from build123d import *

# Parameters (mm, degrees)
SKETCH1_W                      = 120
SKETCH1_H                      = 120
BOSS_EXTRUDE1_DEPTH            = 3
CUT_EXTRUDE1_REACH             = 5
CUT_EXTRUDE1_DIRECTION_2_DEPTH = 1
CUT_EXTRUDE2_REACH             = 5
SKETCH3_R                      = 2.75
SKETCH5_W                      = 124.8
SKETCH5_H                      = 124.8
SKETCH5_W_2                    = 120
SKETCH5_H_2                    = 120
BOSS_EXTRUDE2_DEPTH            = 28
SKETCH6_R                      = 1.65
CUT_EXTRUDE3_DEPTH             = 125.8
SKETCH7_W                      = 4
SKETCH7_H                      = 2
CUT_EXTRUDE4_DEPTH             = 125.8


with BuildPart() as part:
    # Sketch1 → Boss-Extrude1 (new body)
    with BuildSketch(Plane(origin=(0, 0, 0), x_dir=(1, 0, 0), z_dir=(0, 1, 0))):
        with Locations((60, 60)):
            Rectangle(SKETCH1_W, SKETCH1_H)
    extrude(amount=BOSS_EXTRUDE1_DEPTH)

    # Sketch2 → Cut-Extrude1 (cut, up to next)
    with BuildSketch(Plane(origin=(0, 3, 0), x_dir=(1, 0, 0), z_dir=(0, 1, 0)), mode=Mode.PRIVATE) as cut_extrude1_sk1:
        Polygon((15, 115), (57.5, 115), (57.5, 62.5), (5, 62.5), (5, 105), (15, 105), align=None)
    cut_extrude1_tool1 = extrude(cut_extrude1_sk1.sketch, amount=-CUT_EXTRUDE1_REACH, mode=Mode.PRIVATE) & part.part
    add(cut_extrude1_tool1.solids().sort_by_distance((32.05, 3, -87.95))[0], mode=Mode.SUBTRACT)
    # Sketch2 → Cut-Extrude1 (cut, up to next)
    with BuildSketch(Plane(origin=(0, 3, 0), x_dir=(1, 0, 0), z_dir=(0, 1, 0)), mode=Mode.PRIVATE) as cut_extrude1_sk2:
        Polygon((62.5, 5), (62.5, 57.5), (115, 57.5), (115, 15), (105, 15), (105, 5), align=None)
    cut_extrude1_tool2 = extrude(cut_extrude1_sk2.sketch, amount=-CUT_EXTRUDE1_REACH, mode=Mode.PRIVATE) & part.part
    add(cut_extrude1_tool2.solids().sort_by_distance((87.95, 3, -32.05))[0], mode=Mode.SUBTRACT)
    # Sketch2 → Cut-Extrude1 (cut, up to next)
    with BuildSketch(Plane(origin=(0, 3, 0), x_dir=(1, 0, 0), z_dir=(0, 1, 0)), mode=Mode.PRIVATE) as cut_extrude1_sk3:
        Polygon((15, 5), (57.5, 5), (57.5, 57.5), (5, 57.5), (5, 15), (15, 15), align=None)
    cut_extrude1_tool3 = extrude(cut_extrude1_sk3.sketch, amount=-CUT_EXTRUDE1_REACH, mode=Mode.PRIVATE) & part.part
    add(cut_extrude1_tool3.solids().sort_by_distance((32.05, 3, -32.05))[0], mode=Mode.SUBTRACT)
    # Sketch2 → Cut-Extrude1 (cut, up to next)
    with BuildSketch(Plane(origin=(0, 3, 0), x_dir=(1, 0, 0), z_dir=(0, 1, 0)), mode=Mode.PRIVATE) as cut_extrude1_sk4:
        Polygon((115, 62.5), (62.5, 62.5), (62.5, 115), (105, 115), (105, 105), (115, 105), align=None)
    cut_extrude1_tool4 = extrude(cut_extrude1_sk4.sketch, amount=-CUT_EXTRUDE1_REACH, mode=Mode.PRIVATE) & part.part
    add(cut_extrude1_tool4.solids().sort_by_distance((87.95, 3, -87.95))[0], mode=Mode.SUBTRACT)

    # Sketch2 → Cut-Extrude1 direction 2 (cut)
    with BuildSketch(Plane(origin=(0, 3, 0), x_dir=(1, 0, 0), z_dir=(0, 1, 0))):
        Polygon((15, 115), (57.5, 115), (57.5, 62.5), (5, 62.5), (5, 105), (15, 105), align=None)
        Polygon((62.5, 5), (62.5, 57.5), (115, 57.5), (115, 15), (105, 15), (105, 5), align=None)
        Polygon((15, 5), (57.5, 5), (57.5, 57.5), (5, 57.5), (5, 15), (15, 15), align=None)
        Polygon((115, 62.5), (62.5, 62.5), (62.5, 115), (105, 115), (105, 105), (115, 105), align=None)
    extrude(amount=CUT_EXTRUDE1_DIRECTION_2_DEPTH, mode=Mode.SUBTRACT)

    # Sketch3 → Cut-Extrude2 (cut, up to next)
    with BuildSketch(Plane(origin=(0, 3, 0), x_dir=(1, 0, 0), z_dir=(0, 1, 0)), mode=Mode.PRIVATE) as cut_extrude2_sk1:
        with Locations((7.5, 112.5)):
            Circle(SKETCH3_R)
    cut_extrude2_tool1 = extrude(cut_extrude2_sk1.sketch, amount=-CUT_EXTRUDE2_REACH, mode=Mode.PRIVATE) & part.part
    add(cut_extrude2_tool1.solids().sort_by_distance((7.5, 3, -112.5))[0], mode=Mode.SUBTRACT)
    # Sketch3 → Cut-Extrude2 (cut, up to next)
    with BuildSketch(Plane(origin=(0, 3, 0), x_dir=(1, 0, 0), z_dir=(0, 1, 0)), mode=Mode.PRIVATE) as cut_extrude2_sk2:
        with Locations((112.5, 112.5)):
            Circle(SKETCH3_R)
    cut_extrude2_tool2 = extrude(cut_extrude2_sk2.sketch, amount=-CUT_EXTRUDE2_REACH, mode=Mode.PRIVATE) & part.part
    add(cut_extrude2_tool2.solids().sort_by_distance((112.5, 3, -112.5))[0], mode=Mode.SUBTRACT)
    # Sketch3 → Cut-Extrude2 (cut, up to next)
    with BuildSketch(Plane(origin=(0, 3, 0), x_dir=(1, 0, 0), z_dir=(0, 1, 0)), mode=Mode.PRIVATE) as cut_extrude2_sk3:
        with Locations((112.5, 7.5)):
            Circle(SKETCH3_R)
    cut_extrude2_tool3 = extrude(cut_extrude2_sk3.sketch, amount=-CUT_EXTRUDE2_REACH, mode=Mode.PRIVATE) & part.part
    add(cut_extrude2_tool3.solids().sort_by_distance((112.5, 3, -7.5))[0], mode=Mode.SUBTRACT)
    # Sketch3 → Cut-Extrude2 (cut, up to next)
    with BuildSketch(Plane(origin=(0, 3, 0), x_dir=(1, 0, 0), z_dir=(0, 1, 0)), mode=Mode.PRIVATE) as cut_extrude2_sk4:
        with Locations((7.5, 7.5)):
            Circle(SKETCH3_R)
    cut_extrude2_tool4 = extrude(cut_extrude2_sk4.sketch, amount=-CUT_EXTRUDE2_REACH, mode=Mode.PRIVATE) & part.part
    add(cut_extrude2_tool4.solids().sort_by_distance((7.5, 3, -7.5))[0], mode=Mode.SUBTRACT)

    # Sketch5 → Boss-Extrude2 (add)
    with BuildSketch(Plane(origin=(0, 0, 0), x_dir=(1, 0, 0), z_dir=(0, 1, 0))):
        with Locations((60, 60)):
            Rectangle(SKETCH5_W, SKETCH5_H)
        with Locations((60, 60)):
            Rectangle(SKETCH5_W_2, SKETCH5_H_2, mode=Mode.SUBTRACT)
    extrude(amount=BOSS_EXTRUDE2_DEPTH)

    # Sketch6 → Cut-Extrude3 (cut, through all)
    with BuildSketch(Plane.ZY.offset(2.4)):
        with Locations((-112.4, 21)):
            Circle(SKETCH6_R)
        with Locations((-112.4, 7)):
            Circle(SKETCH6_R)
        with Locations((-7.6, 7)):
            Circle(SKETCH6_R)
        with Locations((-7.6, 21)):
            Circle(SKETCH6_R)
    extrude(amount=-CUT_EXTRUDE3_DEPTH, mode=Mode.SUBTRACT)

    # Sketch7 → Cut-Extrude4 (cut, through all)
    with BuildSketch(Plane.ZY.offset(2.4)):
        with Locations((-14.6, 4)):
            Rectangle(SKETCH7_W, SKETCH7_H)
    extrude(amount=-CUT_EXTRUDE4_DEPTH, mode=Mode.SUBTRACT)


solid = part.part
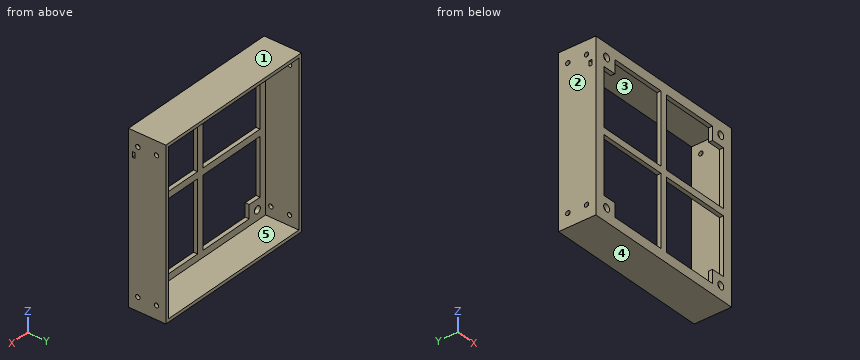
Here's how the part is built. I have some questions about the finished solid (model axes, mm). Face numbers are marked on the shaded views. A direction names the side the tool comes from. Coordinates: 2 decimals unless noted, no trailing zeros. Write each loop counter-clockwise with the first axis right and the second up, starting at its lowest first coordinate (ties: lowest second). Pieces come first, ordered by that corner, then holes.
Item 1: On a 3-axis mill with a long thin cutter (end or side, diameter ignored), from which of +Z, -Z, +X, -X, +Y, -Y can I reach the whole of each face in a straight line? I mean the marked faces 4 and 5. Say none if no direction works.
Item 2: I want a section at A-A on y = 21. Write out the boundary of the cut face in (x, z), and give its area (3 significant figures).
Item 3: If I drill on line 1 (Z direction, x = 7.5, y = 1.45); line 2 (Y direction, x = -1.05, z = -7.6); line 3 (X direction, y = 14, z = -14), over which ranges is the centre line in solid material (lowest first)?
Item 4: I want a section at C-C on x = 17.5. Write out the boundary of the cut face in (y, z), and give its area (3 significant figures).
Item 5: I want a section at D-D on z = -19. Write out the boundary of the cut face in (x, y).
Item 6: If we mould it in two halves opening along Z, with no side actions, what happens to the marked faces 1, 2 and 3? For each: +Z half, -Z half, draft (parallel to the pull), parting line (faces both ways), or undercut.
Item 7: I want a section at B-B on z = -59.5. Write out the boundary of the cut face in (x, y).
Item 8: Will these pins go through, and if not, where does the flat tip stop? pin 1 (6 mm diameter, centred on x = 24.5, z = -57, fed in from +Y); pin 2 (2.5 mm diameter, centred on y = 21, z = -7.6, fed in from -X).
Findings below:
1. face 4: -Z, +X, -X, +Y, -Y
1. face 5: +Y
2. outline: (-2.4, -122.4) - (122.4, -122.4) - (122.4, -114.05) - (120, -114.05) - (120, -120) - (0, -120) - (0, -114.05) - (-2.4, -114.05) - close; (-2.4, -110.75) - (0, -110.75) - (0, -9.25) - (-2.4, -9.25) - close; (-2.4, -5.95) - (0, -5.95) - (0, 0) - (120, 0) - (120, -5.95) - (122.4, -5.95) - (122.4, 2.4) - (-2.4, 2.4) - close; (120, -110.75) - (122.4, -110.75) - (122.4, -9.25) - (120, -9.25) - close
2. area: 1,140 mm2
3. line 1: z = -122.4 to -115.25, -109.75 to -105, -62.5 to -57.5, -15 to -10.25, -4.75 to 2.4
3. line 2: y = 0 to 5.35, 8.65 to 19.35, 22.65 to 28
3. line 3: x = -2.4 to 0, 120 to 122.4
4. outline: (0, -122.4) - (28, -122.4) - (28, -120) - (3, -120) - (3, -115) - (0, -115) - close; (0, -62.5) - (3, -62.5) - (3, -57.5) - (0, -57.5) - close; (0, -5) - (3, -5) - (3, 0) - (28, 0) - (28, 2.4) - (0, 2.4) - close
4. area: 179 mm2
5. outline: (-2.4, 0) - (5, 0) - (5, 3) - (0, 3) - (0, 28) - (-2.4, 28) - close; (57.5, 0) - (62.5, 0) - (62.5, 3) - (57.5, 3) - close; (115, 0) - (122.4, 0) - (122.4, 28) - (120, 28) - (120, 3) - (115, 3) - close
6. face 1: +Z half
6. face 2: draft
6. face 3: undercut
7. outline: (-2.4, 0) - (122.4, 0) - (122.4, 28) - (120, 28) - (120, 3) - (0, 3) - (0, 28) - (-2.4, 28) - close
8. pin 1: stops at y = 3
8. pin 2: passes through
